CAD build for the part. Positions are in the model's coordinates, mm. Face numbers are marked on the shaded views. Coordinates: 2 decimals unless noted, no trailing zeros. Write each loop counter-clockwise with the first axis right and the second up, starting at its lowest first coordinate (ties: lowest second). Pieces come first, ordered by that corner, then holes. Notation, with made-up numbers: (79, 33) -> (118, 33) arc R16 ccw to (118, 42) -> close; hole circle Ø10 at (88.25, 78.5). An arc over 180 degrees is marked (long way). Answer as CSV lines item,"result".
Autodesk Inventor part; units mm, degrees
ref_plane "YZ Plane" through (0, 0, 0) normal (1, 0, 0) x (0, 1, 0)
ref_plane "XZ Plane" through (0, 0, 0) normal (0, 1, 0) x (-1, 0, 0)
ref_plane "XY Plane" through (0, 0, 0) normal (0, 0, 1) x (1, 0, 0)
sketch "Sketch1" plane through (0, 0, 0) normal (0, 0, 1) x (1, 0, 0)
  circle A0 centre (0, 0) radius 13.97
  circle A1 centre (0, 0) radius 19.05
  dimension "d0" = 27.94
  dimension "d1" = 38.1
extrude "Extrusion1" add sketch "Sketch1" along normal blind 100.33
sketch "Sketch2" plane through (0, 0, 0) normal (1, 0, 0) x (0, 1, 0)
  line L0 (-19.05, 100.33) -> (19.05, 100.33)
  line L1 (19.05, 0) -> (19.05, 100.33)
  line L2 (-0.0364, 100.33) -> (-0.0364, 87.2336)
  line L3 (-0.0364, 87.2336) -> (19.05, 82.7907)
  line L4 (-0.0364, 100.33) -> (19.05, 100.33)
  point P0 (0, 0)
extrude "Extrusion2" cut sketch "Sketch2" along normal through all both and the other way through all
chamfer "Chamfer1" distance 6.35 angle 45 2 edges at (16.51, -0.0364, 100.33) (-16.51, -0.0364, 100.33)
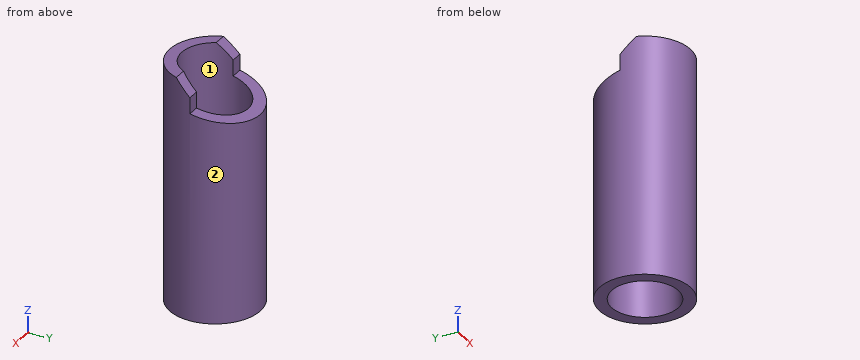
Item 1: Saw through at C-C on z = 81.5. Give the cut face in (x, y).
Answer below:
outline,"circle Ø38.1 at (0, 0); hole circle Ø27.94 at (0, 0)"
Item 2: Two-plate mould, pull along X, no slides. Class the marked faces 1 and 2: pulls with the +X half, pulls with the -X half, needs draft (parallel to the pull), parting line crosses it, or undercut.
Answer below:
face 1,"undercut"
face 2,"parting line crosses it"
Item 3: Saw through at B-B on y = -2. Give the cut face in (x, z).
Answer below:
outline,"(-18.94, 0) -> (-13.83, 0) -> (-13.83, 95.94) -> (-18.94, 95.94) -> close; (13.83, 0) -> (18.94, 0) -> (18.94, 95.94) -> (13.83, 95.94) -> close"
Item 4: Wall check: line 1 (Y direction, x = 0, z = 60.5); line 2 (Y direction, x = 5, z = 46). Give the ranges that are in metal, low to high. Write a range as from..to.
Answer below:
line 1,"y = -19.05..-13.97, 13.97..19.05"
line 2,"y = -18.38..-13.04, 13.04..18.38"
Item 5: Flat gauge pins, fed straight in: pin 1 (1 mm diameter, centred on x = -9, z = 90, fed in from -Y); pin 2 (10 mm diameter, centred on x = -9, z = 19, fed in from -Y); pin 3 (10 mm diameter, centred on y = 13.5, z = 43, fed in from +X); pin 4 (3 mm diameter, centred on x = 13.5, y = 9, fed in from -Z). Where does each tip first touch, or does it go through?
Answer below:
pin 1,"stops at y = -17.05"
pin 2,"stops at y = -18.63"
pin 3,"stops at x = 17.05"
pin 4,"stops at z = 0"
Item 6: Saw through at A-A on x = 0. Give the cut face in (y, z).
Answer below:
outline,"(-19.05, 0) -> (-13.97, 0) -> (-13.97, 100.33) -> (-19.05, 100.33) -> close; (13.97, 0) -> (19.05, 0) -> (19.05, 82.79) -> (13.97, 83.97) -> close"
